```python
from build123d import *

# Parameters (mm, degrees)
PAD_DEPTH       = 13
SKETCH001_R     = 5.5
PAD001_DEPTH    = 15
SKETCH002_R     = 5
POCKET_DEPTH    = 14
SKETCH003_R     = 3
POCKET001_DEPTH = 4.001
SKETCH005_W     = 1
SKETCH005_H     = 3
PAD002_DEPTH    = 4
SKETCH006_W     = 1
SKETCH006_H     = 3
PAD003_DEPTH    = 4
SKETCH007_W     = 2
SKETCH007_H     = 3
PAD004_DEPTH    = 2
SKETCH008_W     = 2
SKETCH008_H     = 3
PAD005_DEPTH    = 2
SKETCH009_R     = 5
SKETCH009_R_2   = 4.5
PAD006_DEPTH    = 13


with BuildPart() as part:
    # Sketch → Pad (new body)
    with BuildSketch(Plane.XY):
        Polygon((-7.5, 1.5), (7.5, 1.5), (8, 11.5), (9, 11.5), (9, -1.5), (-9, -1.5), (-9, 11.5), (-8, 11.5), align=None)
    extrude(amount=PAD_DEPTH)

    # Sketch001 (on Face5 of Pad) → Pad001 (join)
    with BuildSketch(Plane(origin=(0, 1.5, 0), x_dir=(-1, 0, 0), z_dir=(0, 1, 0))):
        with Locations((0, 6.5)):
            Circle(SKETCH001_R)
    extrude(amount=PAD001_DEPTH)

    # Sketch002 (on Face12 of Pad001) → Pocket (cut)
    with BuildSketch(Plane(origin=(0, 16.5, 0), x_dir=(-1, 0, 0), z_dir=(0, 1, 0))):
        with Locations((0, 6.5)):
            Circle(SKETCH002_R)
    extrude(amount=-POCKET_DEPTH, mode=Mode.SUBTRACT)

    # Sketch003 (on Face14 of Pocket) → Pocket001 (cut, through all)
    with BuildSketch(Plane(origin=(0, 2.5, 0), x_dir=(-1, 0, 0), z_dir=(0, 1, 0))):
        with Locations((0, 6.5)):
            Circle(SKETCH003_R)
    extrude(amount=-POCKET001_DEPTH, mode=Mode.SUBTRACT)

    # Sketch005 (on Face8 of Pocket001) → Pad002 (join)
    with BuildSketch(Plane(origin=(0, 11.5, 0), x_dir=(-1, 0, 0), z_dir=(0, 1, 0))):
        with Locations((8.5, 6.5)):
            Rectangle(SKETCH005_W, SKETCH005_H)
    extrude(amount=PAD002_DEPTH)

    # Sketch006 (on Face7 of Pad002) → Pad003 (join)
    with BuildSketch(Plane(origin=(0, 11.5, 0), x_dir=(-1, 0, 0), z_dir=(0, 1, 0))):
        with Locations((-8.5, 6.5)):
            Rectangle(SKETCH006_W, SKETCH006_H)
    extrude(amount=PAD003_DEPTH)

    # Sketch007 (on Face15 of Pad003) → Pad004 (join)
    with BuildSketch(Plane(origin=(-9, 0, 0), x_dir=(0, -1, 0), z_dir=(-1, 0, 0))):
        with Locations((-14.5, 6.5)):
            Rectangle(SKETCH007_W, SKETCH007_H)
    extrude(amount=PAD004_DEPTH)

    # Sketch008 (on Face8 of Pad004) → Pad005 (join)
    with BuildSketch(Plane.YZ.offset(9)):
        with Locations((14.5, 6.5)):
            Rectangle(SKETCH008_W, SKETCH008_H)
    extrude(amount=PAD005_DEPTH)

    # Sketch009 (on Face16 of Pad005) → Pad006 (join)
    with BuildSketch(Plane(origin=(0, 2.5, 0), x_dir=(-1, 0, 0), z_dir=(0, 1, 0))):
        with Locations((0, 6.5)):
            Circle(SKETCH009_R)
        with Locations((0, 6.5)):
            Circle(SKETCH009_R_2, mode=Mode.SUBTRACT)
    extrude(amount=PAD006_DEPTH)


solid = part.part
```
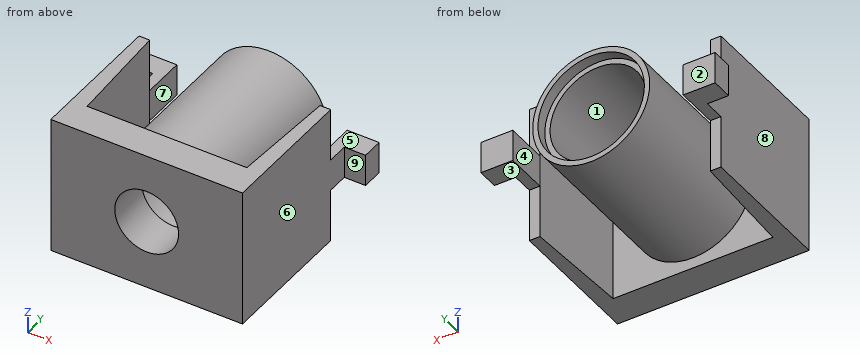
For this review, take the finished solid that the model builds, in its own axes (mm). Face numbers are marked on the shaded views. A direction names the side the tool comes from. Coordinates: 2 decimals unless noted, no trailing zeros. Write each loop counter-clockwise with the first axis right and the second up, starting at its lowest first coordinate (ties: lowest second). Pieces come first, ordered by that corner, then holes.
(1) Wall thickness on probe 1 along X at (y, z) = (11, 4) (3 decimals); probe 2 along Z at (x, y) = (0, 16.15); probe 3 along Z at (x, y) = (0, 14.5): over which ranges is each line inside the solid? List them lowest first.
(2) For pin 1 Ø3.5 at (x, y) = (9.5, 14.5) entering from -Z; pin 2 Ø1.5 at (y, z) = (10.5, 3) entering from -X; pin 3 Ø1 at (y, z) = (2, 5.5) entering from +X, all flat-tipped, find the tip position at first contact; note any pin that passes through.
(3) Add section D-D on y = 14.75. Give the boundary of the cut face in (x, z).
(4) Tool access review of the marked faces 1, 2, 3, 4 and 5: name each direction out of +Z, -Z, +X, -X, +Y, -Y from which nothing blocks a thin tool from reaching the whole face with its end or side.
(5) The part is to be moulded in two halves that separate along X. For the marked faces 6, 7, 8 and 9, say which applies: +X half, -X half, draft (parallel to the pull), parting line (faces both ways), or undercut.
(6) Add section A-A on y = 3.5. Give the boundary of the cut face in (x, z).
(7) Add section C-C on x = 0. Give the boundary of the cut face in (y, z).
Answer sheet:
1. probe 1: x = -9 to -7.975, -4.899 to -3.742, 3.742 to 4.899, 7.975 to 9
1. probe 2: z = 1 to 1.5, 11.5 to 12
1. probe 3: z = 1 to 2, 11 to 12
2. pin 1: stops at z = 5
2. pin 2: stops at x = -9
2. pin 3: stops at x = 9
3. outline: (-11, 5) - (-8, 5) - (-8, 8) - (-11, 8) - close; circle Ø11 at (0, 6.5); (8, 5) - (11, 5) - (11, 8) - (8, 8) - close; hole circle Ø9 at (0, 6.5)
4. face 1: +Y
4. face 2: +Z, -Z, -X, +Y
4. face 3: -Z, +X, +Y
4. face 4: +Z, -Z, +Y
4. face 5: +Z, +X, +Y
5. face 6: +X half
5. face 7: undercut
5. face 8: -X half
5. face 9: draft
6. outline: (-9, 0) - (-7.6, 0) - (-7.6, 13) - (-9, 13) - close; circle Ø11 at (0, 6.5); (7.6, 0) - (9, 0) - (9, 13) - (7.6, 13) - close; hole circle Ø9 at (0, 6.5)
7. outline: (-1.5, 0) - (1.5, 0) - (1.5, 1) - (16.5, 1) - (16.5, 1.5) - (15.5, 1.5) - (15.5, 2) - (2.5, 2) - (2.5, 3.5) - (-1.5, 3.5) - close; (-1.5, 9.5) - (2.5, 9.5) - (2.5, 11) - (15.5, 11) - (15.5, 11.5) - (16.5, 11.5) - (16.5, 12) - (1.5, 12) - (1.5, 13) - (-1.5, 13) - close
